```python
from build123d import *

# Parameters (mm, degrees)
SKETCH1_R               = 6
BOSS_EXTRUDE1_DEPTH     = 50
CUT_EXTRUDE2_START      = 50
SKETCH1_4_R             = 4.05
CUT_EXTRUDE2_DEPTH      = 15
SKETCH3_R               = 1.5
CUT_EXTRUDE3_DEPTH      = 7
CUT_EXTRUDE3_DEPTH_BACK = 7


with BuildPart() as part:
    # Sketch1 → Boss-Extrude1 (new body)
    with BuildSketch(Plane(origin=(0, 0, 0), x_dir=(1, 0, 0), z_dir=(0, 1, 0))):
        Circle(SKETCH1_R)
    extrude(amount=BOSS_EXTRUDE1_DEPTH)

    # Sketch1<4> → Cut-Extrude2 (cut)
    with BuildSketch(Plane(origin=(0, 0, 0), x_dir=(1, 0, 0), z_dir=(0, 1, 0)).offset(CUT_EXTRUDE2_START)):
        Circle(SKETCH1_4_R)
    extrude(amount=-CUT_EXTRUDE2_DEPTH, mode=Mode.SUBTRACT)

    # Sketch3 → Cut-Extrude3 (cut, two sides)
    with BuildSketch(Plane.XY) as cut_extrude3_sk:
        with Locations((0, 7.20619719)):
            Circle(SKETCH3_R)
    extrude(amount=CUT_EXTRUDE3_DEPTH, mode=Mode.SUBTRACT)
    extrude(cut_extrude3_sk.sketch, amount=-CUT_EXTRUDE3_DEPTH_BACK, mode=Mode.SUBTRACT)


solid = part.part
```
Read the model definition and answer for the solid it produces. Units are mm, in the model's axes. A direction names the side the tool comes from. Round coordinates to 2 decimals unless told otherwise and drop trailing zeros. Write each loop counter-clockwise with the first axis right and the second up, starting at its lowest first coordinate (ties: lowest second). Pieces come first, ordered by that corner, then holes. Notation, with made-up numbers: (69, -34.75) - (115, -34.75) arc R17 ccw to (115, -20.75) - close; hole circle Ø8 at (29.5, 87.25). An arc over 180 degrees is marked (long way). Use CSV: the item, a comma, the result in double quotes.
Q1. Each of these flat-tipped pins is pushed along its axis until it touches: pin 1 Ø4 at (y, z) = (39, 3.5) entering from -X; pin 2 Ø5 at (x, y) = (4, 41.5) entering from -Z; pin 3 Ø5 at (x, y) = (-3.5, 32) entering from +Z. Where does it stop, or does it pass through?
Values:
pin 1,"stops at x = -5.81"
pin 2,"stops at z = -5.81"
pin 3,"stops at z = 5.92"
Q2. Straight lines are drawn through the part: line 1 along Y through (x, z) = (0, 3.25); line 2 along Y through (x, z) = (0, -4.25); line 3 along X through (y, z) = (8, -0.5). For each, find the intervals that lie inside material, in ascending order.
Values:
line 1,"y = 0 to 5.71, 8.71 to 35"
line 2,"y = 0 to 5.71, 8.71 to 50"
line 3,"x = -5.98 to -1.27, 1.27 to 5.98"
Q3. Find section D-D, the plane x = -2. Write down the section's boundary in (y, z).
Values:
outline,"(0, -5.66) - (50, -5.66) - (50, -3.52) - (35, -3.52) - (35, 3.52) - (50, 3.52) - (50, 5.66) - (0, 5.66) - close"
Q4. Find section B-B, the plane z = 0. Write down the section's boundary in (x, y).
Values:
outline,"(-6, 0) - (6, 0) - (6, 50) - (4.05, 50) - (4.05, 35) - (-4.05, 35) - (-4.05, 50) - (-6, 50) - close; hole circle Ø3 at (0, 7.21)"
Q5. A tool of negligible diameter and unlimited length cuts with its end or side. For faces 4 (the cylindrical face through (-0.195, 8.693, 0.084)), 5 (the cylindrical face through (-0.878, 42.605, 3.954)), from which of +Z, -Z, +X, -X, +Y, -Y can it reach the whole face along a straight path? Write none if from no direction.
Values:
face 4,"+Z, -Z"
face 5,"+Y"
Q6. Determine the mould class of faces 1 (the flat face through (0, 0, 0)), 2 (the flat face through (0, 35, 0)), 3 (the cylindrical face through (-1.301, 24.65, 5.857)) for opening direction X: +X half, -X half, draft (parallel to the pull), parting line (faces both ways), or undercut.
Values:
face 1,"draft"
face 2,"undercut"
face 3,"parting line"
Q7. Find section C-C, the plane y = 40.5. Write down the section's boundary in (x, z), then the cut area to 3 significant figures.
Values:
outline,"circle Ø12 at (0, 0); hole circle Ø8.1 at (0, 0)"
area,"61.6 mm²"
Q8. Find section A-A, the plane x = 0. Write down the section's boundary in (y, z), then the cut area to 4 significant figures.
Values:
outline,"(0, -6) - (5.71, -6) - (5.71, 6) - (0, 6) - close; (8.71, -6) - (50, -6) - (50, -4.05) - (35, -4.05) - (35, 4.05) - (50, 4.05) - (50, 6) - (8.71, 6) - close"
area,"442.5 mm²"
